Check sheet for the modelled part. Datum: model origin and axes. Units: mm. Face numbers are marked on the shaded views. Round coordinates to 2 decimals unless told otherwise and drop trailing zeros. Order: outer loops, then holes, each group sorted by start corner. A loop starts at its lowest first (then second) coordinate and runs counter-clockwise, first axis right, second up.
(1) Mould release check, pull along Z, two halves, no side actions. Record for the marked faces 1 and 2: released by +Z, released by -Z, zero draft, split by the parting line, or undercut.
(2) Sectioned sample at C-C, the plane x = 61. Enter the section's corners in (y, z).
(3) Thickness scan on probe 1 along Y at (x, z) = (210, 15.5); probe 2 along Z at (x, y) = (11, 148.5); probe 3 along Y at (x, z) = (-172, 1). Record the ranges inside material, lowest first.
(4) Sectioned sample at D-D, the plane y = 0. Count the separate pieces of the cut face and the enclosed holes in it, and give its area (3 significant figures).
(5) Sectioned sample at B-B, the plane y = 92.5. Enter the section's corners in (x, z).
(6) Depth check by flat-ended pin: pin 1 (6 mm diameter, centred on y = 6.5, z = 4.5, fed in from +X); pin 2 (9.5 mm diameter, centred on x = 210, y = -1.5, fed in from -Z); pin 3 (24 mm diameter, centred on x = -44, y = 1.5, fed in from +Z). Enter the tip coordinate at first touch or a pass-through.
(7) Sectioned sample at A-A, the plane x = -93.5. Enter the section's corners in (y, z).
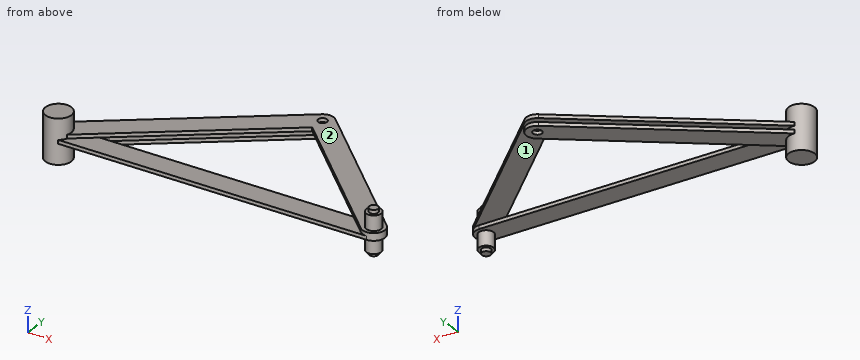
```python
from build123d import *

# Parameters (mm, degrees)
SKETCH_1_W      = 450
SKETCH_1_H      = 30
EXTRUDE_1_DEPTH = 5
FILLET_1_RADIUS = 15
FILLET_1_LENGTH = 5
FILLET_2_RADIUS = 15
FILLET_2_LENGTH = 5
SKETCH_2_R      = 10
SKETCH_2_R_2    = 6
EXTRUDE_2_DEPTH = 17.5
SKETCH_4_R      = 6
EXTRUDE_3_DEPTH = 5
SKETCH_5_R      = 6
EXTRUDE_4_DEPTH = 5
EXTRUDE_START   = 7.5
SKETCH_6_R      = 10
EXTRUDE_5_DEPTH = 7.5
SKETCH_7_R      = 6
EXTRUDE_6_DEPTH = 5
SKETCH_8_R      = 17.5
EXTRUDE_7_DEPTH = 30


with BuildPart() as part:
    # 草图1 → 凸台-拉伸1 (new body)
    with BuildSketch(Plane.XY):
        Rectangle(SKETCH_1_W, SKETCH_1_H)
    extrude(amount=EXTRUDE_1_DEPTH)

    # 圆角1: full round fillet: the end face becomes a half cylinder, R = half its width
    fillet_1_face = Plane((-225, 0, 2.5), x_dir=(0, 0, 1), z_dir=(-1, 0, 0))  # on the end face: x along it, z out of the body
    fillet_1_slab = fillet_1_face.offset(-FILLET_1_RADIUS / 2) * Box(FILLET_1_LENGTH, 2 * FILLET_1_RADIUS, FILLET_1_RADIUS, mode=Mode.PRIVATE)  # the body's end, R deep
    fillet_1_round = Plane((-210, 0, 2.5), x_dir=(-1, 0, 0), z_dir=(0, 0, 1)) * Cylinder(FILLET_1_RADIUS, FILLET_1_LENGTH, mode=Mode.PRIVATE)  # its axis R under the face
    add(fillet_1_slab - fillet_1_round, mode=Mode.SUBTRACT)

    # 圆角2: full round fillet: the end face becomes a half cylinder, R = half its width
    fillet_2_face = Plane((225, 0, 2.5), x_dir=(0, 0, -1), z_dir=(1, 0, 0))  # on the end face: x along it, z out of the body
    fillet_2_slab = fillet_2_face.offset(-FILLET_2_RADIUS / 2) * Box(FILLET_2_LENGTH, 2 * FILLET_2_RADIUS, FILLET_2_RADIUS, mode=Mode.PRIVATE)  # the body's end, R deep
    fillet_2_round = Plane((210, 0, 2.5), x_dir=(1, 0, 0), z_dir=(0, 0, -1)) * Cylinder(FILLET_2_RADIUS, FILLET_2_LENGTH, mode=Mode.PRIVATE)  # its axis R under the face
    add(fillet_2_slab - fillet_2_round, mode=Mode.SUBTRACT)

    # 草图2 → 凸台-拉伸2 (add, symmetric)
    # profile 1 of 2: a face of its own
    with BuildSketch(Plane.XY.offset(5)):
        with Locations(Location((-215, 0, 0), (0, 0, 180.000443811))):
            Circle(SKETCH_2_R)
        with Locations((-215, 0)):
            Circle(SKETCH_2_R_2, mode=Mode.SUBTRACT)
    # profile 2 of 2: a face of its own
    with BuildSketch(Plane.XY.offset(5)):
        with Locations((210, 0)):
            Circle(SKETCH_2_R)
        with Locations((210, 0)):
            Circle(SKETCH_2_R_2, mode=Mode.SUBTRACT)
    extrude(amount=EXTRUDE_2_DEPTH, both=True)

    # 草图4 → 凸台-拉伸3 (add)
    with BuildSketch(Plane.XY.offset(5)):
        with BuildLine():
            Line((199.561031329, -10.771626298), (16.443384271, 166.690841102))
            ThreePointArc((16.443384271, 166.690841102), (16.110726644, 187.90143607), (37.321321612, 188.234093697))
            Line((37.321321612, 188.234093697), (220.438968671, 10.771626298))
            ThreePointArc((220.438968671, 10.771626298), (220.771626298, -10.438968671), (199.561031329, -10.771626298))
        make_face()
        with Locations((26.882352941, 177.4624674)):
            Circle(SKETCH_4_R, mode=Mode.SUBTRACT)
    extrude(amount=EXTRUDE_3_DEPTH)

    # 草图5 → 凸台-拉伸4 (add)
    with BuildSketch(Plane.XY.offset(5)):
        with BuildLine():
            Line((-223.87312337, 12.094117647), (18.009229571, 189.556585047))
            ThreePointArc((18.009229571, 189.556585047), (38.976470588, 186.33559077), (35.755476311, 165.368349753))
            Line((35.755476311, 165.368349753), (-206.12687663, -12.094117647))
            ThreePointArc((-206.12687663, -12.094117647), (-227.094117647, -8.87312337), (-223.87312337, 12.094117647))
        make_face()
        with Locations((26.882352941, 177.4624674)):
            Circle(SKETCH_5_R, mode=Mode.SUBTRACT)
    extrude_4 = extrude(amount=EXTRUDE_4_DEPTH)

    # 镜向1: 凸台-拉伸4 across plane
    add(extrude_4.mirror(Plane.XY.offset(2.5)))

    # 草图6 → 凸台-拉伸5 (add)
    with BuildSketch(Plane.XY.offset(22.5).offset(EXTRUDE_START)):
        with Locations((210, 0)):
            Circle(SKETCH_6_R)
    extrude_5 = extrude(amount=-EXTRUDE_5_DEPTH)

    # 草图7 → 凸台-拉伸6 (add)
    with BuildSketch(Plane.XY.offset(30)):
        with Locations((210, 0)):
            Circle(SKETCH_7_R)
    extrude_6 = extrude(amount=EXTRUDE_6_DEPTH)

    # 镜向2: 凸台-拉伸5, 凸台-拉伸6 across plane
    add(extrude_5.mirror(Plane.XY.offset(5)))
    add(extrude_6.mirror(Plane.XY.offset(5)))

    # 草图8 → 凸台-拉伸7 (add, symmetric)
    with BuildSketch(Plane.XY.offset(2.5)):
        with Locations((-215, 0)):
            Circle(SKETCH_8_R)
    extrude(amount=EXTRUDE_7_DEPTH, both=True)


solid = part.part
```
Derived:
1. face 1: undercut
1. face 2: released by +Z
2. outline: (-15, 0) - (15, 0) - (15, 5) - (-15, 5) - close; (123.51, 5) - (165.29, 5) - (165.29, 10) - (123.51, 10) - close
3. probe 1: y = -10 to -6, 6 to 10
3. probe 2: z = -5 to 0, 5 to 10
3. probe 3: y = -15 to 15
4. separate pieces: 1
4. enclosed holes: 2
4. area: 5,090 mm2
5. outline: (-114.28, -5) - (-63.56, -5) - (-63.56, 0) - (-114.28, 0) - close; (-114.28, 5) - (-63.56, 5) - (-63.56, 10) - (-114.28, 10) - close; (93, 5) - (136.11, 5) - (136.11, 10) - (93, 10) - close
6. pin 1: stops at x = 224.59
6. pin 2: stops at z = -25
6. pin 3: stops at z = 5
7. outline: (-15, 0) - (15, 0) - (15, 5) - (-15, 5) - close; (70.54, -5) - (107.75, -5) - (107.75, 0) - (70.54, 0) - close; (70.54, 5) - (107.75, 5) - (107.75, 10) - (70.54, 10) - close
